Solid Edge part; units mm, degrees
sketch "Sketch1" plane through (0, 0, 0) normal (0, 0, 1) x (1, 0, 0)
  circle A0 centre (0, 0) radius 46.5
extrude "Protrusion1" add sketch "Sketch1" along normal blind 3
sketch "Sketch2" plane through (0, 0, 0) normal (0, 0, 1) x (1, 0, 0)
  circle A0 centre (0, 0) radius 46.5
  circle A1 centre (0, 0) radius 44.5
extrude "ExtrudedProtrusion_4" add sketch "Sketch2" along normal blind 10
sketch "Sketch3" plane through (0, 0, 0) normal (0, 0, 1) x (1, 0, 0)
  line L0 (35.8, -19.5) -> (35.8, 19.3)
  line L1 (35.8, 19.3) -> (18, 19.3)
  line L2 (18, 19.3) -> (18, -19.5)
  line L3 (18, -19.5) -> (35.8, -19.5)
extrude "ExtrudedCutout_2" cut sketch "Sketch3" along normal blind 2
sketch "Sketch4" plane through (0, 0, 0) normal (0, 0, 1) x (1, 0, 0)
  circle A0 centre (0, 0) radius 14.25
extrude "Cutout1" cut sketch "Sketch4" along normal through all
chamfer "Chamfer_1" distance 1 angle 45 1 edges at (-46.5, 0, 10) measured on face at (-31.93, 31.93, 10)
The model under review builds one solid part; all positions refer to its coordinate system, in mm. A direction names the side the tool comes from. Round coordinates to 2 decimals unless told otherwise and drop trailing zeros. Loops run counter-clockwise (first coordinate to the right, second up) from the corner with the lowest first, then second, coordinate; pieces in that order, holes last. Notation, with made-up numbers: (52.25, -20.75) -> (74.25, -20.75) arc R10 cw to (74.25, -13.75) -> close; hole circle Ø11 at (8, -26.5). An arc over 180 degrees is marked (long way). Answer as a JSON object with one key per item and string values. Group by question number.
1) For faces 1 (the face through (27, 19.3, 1)), 2 (the face through (-32.798, -30.075, 6.451)), 3 (the face through (10, -44, 10)), list the 3-axis set-ups (+Z, -Z, +X, -X, +Y, -Y) from which the entire face can be reached by the end or side of a thin tool; tool diameter is ignored.
2) We need section C-C on z = 5.25. Write out the cut boundary in (x, y), then the cut area to 3 significant figures.
3) We need section A-A on x = 0. Write out the cut boundary in (y, z).
4) For line 1 (Y direction, x = 0, z = 1.25); line 2 (Y direction, x = 0, z = 7.5); line 3 (Z direction, x = -39, y = -4), list the stretches that pass through material, from the lowest coordinate up. Write a range as [from, to].
5) For pin 1 Ø2 at (x, y) = (-36, -0.5) entering from -Z; pin 2 Ø6 at (x, y) = (-21.5, -20.5) entering from +Z; pin 3 Ø1.6 at (y, z) = (2, 1) entering from -X; pin 4 Ø0.6 at (y, z) = (-2.5, 1.5) entering from +X, all flat-tipped, find the tip position at first contact; note any pin that passes through.
6) We need section B-B on y = 0. Write out the cut boundary in (x, z).
Result set:
{
 "1": {"face 1": "-Z", "face 2": "+Z", "face 3": "+Z, +X, -X, +Y, -Y"},
 "2": {"outline": "circle Ø93 at (0, 0); hole circle Ø89 at (0, 0)", "area": "572 mm²"},
 "3": {"outline": "(-46.5, 0) -> (-14.25, 0) -> (-14.25, 3) -> (-44.5, 3) -> (-44.5, 10) -> (-45.5, 10) -> (-46.5, 9) -> close; (14.25, 0) -> (46.5, 0) -> (46.5, 9) -> (45.5, 10) -> (44.5, 10) -> (44.5, 3) -> (14.25, 3) -> close"},
 "4": {"line 1": "[-46.5, -14.25], [14.25, 46.5]", "line 2": "[-46.5, -44.5], [44.5, 46.5]", "line 3": "[0, 3]"},
 "5": {"pin 1": "z = 0", "pin 2": "z = 3", "pin 3": "x = -46.48", "pin 4": "x = 46.45"},
 "6": {"outline": "(-46.5, 0) -> (-14.25, 0) -> (-14.25, 3) -> (-44.5, 3) -> (-44.5, 10) -> (-45.5, 10) -> (-46.5, 9) -> close; (14.25, 0) -> (18, 0) -> (18, 2) -> (35.8, 2) -> (35.8, 0) -> (46.5, 0) -> (46.5, 9) -> (45.5, 10) -> (44.5, 10) -> (44.5, 3) -> (14.25, 3) -> close"}
}
